Geometry check sheet. Reference: the model listing, model coordinates, mm. A direction names the side the tool comes from. Give positions to 0.01 mm unless a question says otherwise; leave off trailing zeros. Write each loop counter-clockwise with the first axis right and the second up, starting at its lowest first coordinate (ties: lowest second). Pieces come first, ordered by that corner, then holes. Notation, with made-up numbers: (50.25, 28.25) - (93.25, 28.25) arc R21 cw to (93.25, 36.25) - close; hole circle Ø1 at (81, 19.5). An arc over 180 degrees is marked (long way). Write item = value, one per line. Start each with the question number.
(1) Access from +Z, -Z, +X, -X, +Y, -Y to the whole of each face (thin tool, end or side, straight path). Record for faces 4 (the flat face through (-1, -3, -22)), 5 (the flat face through (-11.35, -12.93, -3.57)), 6 (the cylindrical face through (-3.91, -13.07, 12.36)).
(2) Section check A-A, the plane y = -16.5. Enter the section's corners in (x, z), plus the area to 3 significant figures.
(3) Thickness scan on L1, parallel to Y at x = 16.5, z = 21; L2, parallel to Z at x = 0, y = -8.75; L3, parallel to Z at x = 4, y = -19.25. Record the ranges inside material, lowest first.
(4) Draft check along X on faces 1 (the cylindrical face through (-0.59, -11.34, 4.46)), 2 (the cylindrical face through (7.73, -21.574, -6.949)), 3 (the flat face through (-4, -23, -3)). Enter one of: pulls with the +X half, pulls with the -X half, needs draft (parallel to the pull), parting line crosses it, or undercut.
```python
from build123d import *

# Parameters (mm, degrees)
F0_R     = 50.1
F0_R_2   = 4.5
F1_DEPTH = 3
F2_R     = 4.5
F3_DEPTH = 20
F4_R     = 2.99999
F5_R     = 5
F6_R     = 5


# Not quite as in the source:
# - a fillet or chamfer is up to 0.001 mm smaller than in the source, because OpenCascade refuses the exact size


with BuildPart() as f1:
    # F0 (on Front) → F1 (new body)
    with BuildSketch(Plane.XZ):
        Circle(F0_R)
        Circle(F0_R_2, mode=Mode.SUBTRACT)
    extrude(amount=F1_DEPTH)

    # F2 (on face) → F3 (join)
    with BuildSketch(Plane.XZ.offset(3)):
        Polygon((9.2398859849, 10.167053197), (-4.1849833578, 13.0855025895), (-13.4248693427, 2.9184493925), (-9.2398859849, -10.167053197), (4.1849833578, -13.0855025895), (13.4248693427, -2.9184493925), align=None)
        Circle(F2_R, mode=Mode.SUBTRACT)
    extrude(amount=F3_DEPTH)

    # F4 (radius 3 in the source; OpenCascade refuses exactly that, so slightly less here)
    f4_edges = [f1.edges().sort_by_distance(p)[0] for p in [
        (-50.1, 0, 0),
    ]]
    fillet(f4_edges, radius=F4_R)

    # F5
    f5_edges = [f1.edges().sort_by_distance(p)[0] for p in [
        (-4.184983, -13, 13.085503),
        (9.239886, -13, 10.167053),
        (13.424869, -13, -2.918449),
        (4.184983, -13, -13.085503),
        (-9.239886, -13, -10.167053),
        (-13.424869, -13, 2.918449),
    ]]
    fillet(f5_edges, radius=F5_R)

    # F6
    f6_edges = [f1.edges().sort_by_distance(p)[0] for p in [
        (11.332378, -3, 3.624302),
        (12.545511, -13, -0.168893),
        (10.119245, -13, 7.417497),
        (11.332378, -23, 3.624302),
    ]]
    fillet(f6_edges, radius=F6_R)


solid = f1.part
```
Model answer:
q1.face_4 = -Y
q1.face_5 = -Z, -X, -Y
q1.face_6 = +Z, -Y
q2.outline = (-12.55, 0.17) - (-10.12, -7.42) arc R5 ccw to (-6.42, -10.78) - (1.36, -12.47) arc R5 ccw to (6.13, -10.95) - (11.48, -5.05) arc R5 ccw to (12.55, -0.17) - (10.12, 7.42) arc R5 ccw to (6.42, 10.78) - (-1.36, 12.47) arc R5 ccw to (-6.13, 10.95) - (-11.48, 5.05) arc R5 ccw to start; hole circle Ø9 at (0, 0)
q2.area = 419 mm²
q3.L1 = -3 to 0
q3.L2 = -12.18 to -4.5, 4.5 to 12.18
q3.L3 = -12.16 to -2.06, 2.06 to 11.14
q4.face_1 = undercut
q4.face_2 = pulls with the +X half
q4.face_3 = needs draft
